Geometry: final body of the model. Coordinates: model frame, mm. Face numbers are marked on the shaded views. A direction names the side the tool comes from. Coordinates: 2 decimals unless noted, no trailing zeros. Order: outer loops, then holes, each group sorted by start corner. A loop starts at its lowest first (then second) coordinate and runs counter-clockwise, first axis right, second up. Notation, with made-up numbers: (38.25, 55) - (95.25, 55) arc R19 cw to (95.25, 71) - close; hole circle Ø2 at (7, 62.25). An arc over 180 degrees is marked (long way). Use a Markdown table: item, result. Add a question column.
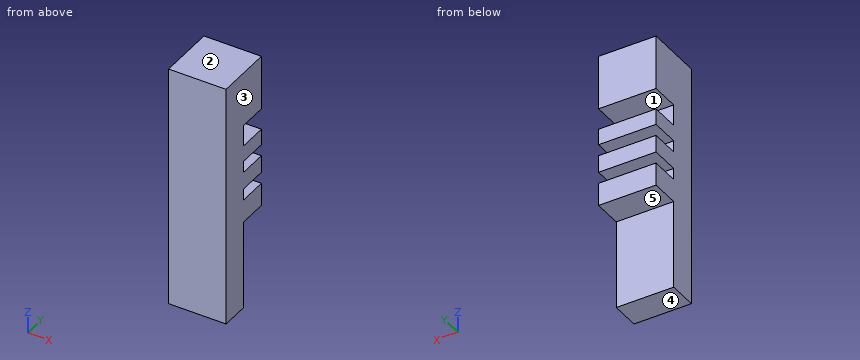
```python
from build123d import *

# Parameters (mm, degrees)
SKETCH1_W           = 10
SKETCH1_H           = 42.5
BOSS_EXTRUDE1_DEPTH = 5
SKETCH2_W           = 10
SKETCH2_H           = 4
BOSS_EXTRUDE2_DEPTH = 5


with BuildPart() as part:
    # Sketch1 → Boss-Extrude1 (new body)
    with BuildSketch(Plane(origin=(0, 0, 0), x_dir=(1, 0, 0), z_dir=(0, 1, 0))):
        with Locations((5, 21.25)):
            Rectangle(SKETCH1_W, SKETCH1_H)
    extrude(amount=BOSS_EXTRUDE1_DEPTH)

    # Sketch2 → Boss-Extrude2 (add)
    with BuildSketch(Plane(origin=(0, 5, 0), x_dir=(1, 0, 0), z_dir=(0, 1, 0))):
        with BuildLine():
            Line((0, 9.5), (0, 0))
            Line((0, 0), (10, 0))
            Line((10, 0), (10, 9.5))
            Line((10, 9.5), (6.38985528, 9.5))
            add(Edge.make_bspline(
                [(6.38985528, 9.5), (6.385913474, 9.499063167), (6.369337183, 9.495284951), (6.339528779, 9.489593982), (6.299971793, 9.48472811), (6.259281687, 9.481095847), (6.231779336, 9.480879047), (6.217848558, 9.480769231)],
                knots=[11.350502485, 11.350502485, 11.350502485, 11.350502485, 11.676244097, 12.717260333, 13.78922464, 14.880174919, 16, 16, 16, 16], degree=3))
            add(Edge.make_bspline(
                [(6.217848558, 9.480769231), (6.19658675, 9.481151208), (6.154913454, 9.481899886), (6.098774023, 9.489476712), (6.064160656, 9.496513578), (6.049680169, 9.5)],
                knots=[0, 0, 0, 0, 1.1129367, 2.181364009, 2.961379824, 2.961379824, 2.961379824, 2.961379824], degree=3))
            Line((6.049680169, 9.5), (5.326923077, 9.5))
            Line((5.326923077, 9.5), (5.192307692, 9.5))
            Line((5.192307692, 9.5), (4.903846154, 9.5))
            Line((4.903846154, 9.5), (4.769230769, 9.5))
            Line((4.769230769, 9.5), (4.12352071, 9.5))
            Line((4.12352071, 9.5), (3.942307692, 9.096153846))
            Line((3.942307692, 9.096153846), (3.796875, 9.096153846))
            Line((3.796875, 9.096153846), (3.978178742, 9.5))
            Line((3.978178742, 9.5), (3.173076923, 9.5))
            Line((3.173076923, 9.5), (3.038461538, 9.5))
            Line((3.038461538, 9.5), (2.466778357, 9.5))
            add(Edge.make_bspline(
                [(2.466778357, 9.5), (2.462836551, 9.499063167), (2.44626026, 9.495284951), (2.416451856, 9.489593982), (2.37689487, 9.48472811), (2.336204764, 9.481095847), (2.308702413, 9.480879047), (2.294771635, 9.480769231)],
                knots=[11.350502485, 11.350502485, 11.350502485, 11.350502485, 11.676244097, 12.717260333, 13.78922464, 14.880174919, 16, 16, 16, 16], degree=3))
            add(Edge.make_bspline(
                [(2.294771635, 9.480769231), (2.273509827, 9.481151208), (2.231836531, 9.481899886), (2.1756971, 9.489476712), (2.141083733, 9.496513578), (2.126603246, 9.5)],
                knots=[0, 0, 0, 0, 1.1129367, 2.181364009, 2.961379824, 2.961379824, 2.961379824, 2.961379824], degree=3))
            Line((2.126603246, 9.5), (1.5, 9.5))
            Line((1.5, 9.5), (1.353665865, 9.5))
            Line((1.353665865, 9.5), (0.223858173, 9.5))
            Line((0.223858173, 9.5), (0.076923077, 9.5))
            Line((0.076923077, 9.5), (0, 9.5))
        make_face()
        with BuildLine():
            add(Edge.make_bspline(
                [(6.38985528, 9.5), (6.385913474, 9.499063167), (6.369337183, 9.495284951), (6.339528779, 9.489593982), (6.299971793, 9.48472811), (6.259281687, 9.481095847), (6.231779336, 9.480879047), (6.217848558, 9.480769231)],
                knots=[11.350502485, 11.350502485, 11.350502485, 11.350502485, 11.676244097, 12.717260333, 13.78922464, 14.880174919, 16, 16, 16, 16], degree=3))
            Line((6.38985528, 9.5), (6.049680169, 9.5))
            add(Edge.make_bspline(
                [(6.217848558, 9.480769231), (6.19658675, 9.481151208), (6.154913454, 9.481899886), (6.098774023, 9.489476712), (6.064160656, 9.496513578), (6.049680169, 9.5)],
                knots=[0, 0, 0, 0, 1.1129367, 2.181364009, 2.961379824, 2.961379824, 2.961379824, 2.961379824], degree=3))
        make_face()
        with BuildLine():
            Line((2.466778357, 9.5), (2.126603246, 9.5))
            add(Edge.make_bspline(
                [(2.294771635, 9.480769231), (2.273509827, 9.481151208), (2.231836531, 9.481899886), (2.1756971, 9.489476712), (2.141083733, 9.496513578), (2.126603246, 9.5)],
                knots=[0, 0, 0, 0, 1.1129367, 2.181364009, 2.961379824, 2.961379824, 2.961379824, 2.961379824], degree=3))
            add(Edge.make_bspline(
                [(2.466778357, 9.5), (2.462836551, 9.499063167), (2.44626026, 9.495284951), (2.416451856, 9.489593982), (2.37689487, 9.48472811), (2.336204764, 9.481095847), (2.308702413, 9.480879047), (2.294771635, 9.480769231)],
                knots=[11.350502485, 11.350502485, 11.350502485, 11.350502485, 11.676244097, 12.717260333, 13.78922464, 14.880174919, 16, 16, 16, 16], degree=3))
        make_face()
        Polygon((3.942307692, 9.096153846), (4.12352071, 9.5), (3.978178742, 9.5), (3.796875, 9.096153846), align=None)
        with BuildLine():
            Line((0, 21), (0, 18))
            Line((0, 18), (10, 18))
            Line((10, 18), (10, 21))
            Line((10, 21), (4.598525657, 21))
            add(Edge.make_bspline(
                [(4.598525657, 21), (4.598135805, 20.999899395), (4.580997325, 20.995497464), (4.545939577, 20.988338664), (4.491951793, 20.98190012), (4.454946287, 20.981152202), (4.435997596, 20.980769231)],
                knots=[8.84081453, 8.84081453, 8.84081453, 8.84081453, 8.864066838, 9.862729781, 10.905609505, 12, 12, 12, 12], degree=3))
            add(Edge.make_bspline(
                [(4.435997596, 20.980769231), (4.414936749, 20.981260877), (4.373853136, 20.982219937), (4.320342805, 20.98961816), (4.288253752, 20.996770904), (4.275833044, 21)],
                knots=[0, 0, 0, 0, 1.145258523, 2.234067595, 2.931969346, 2.931969346, 2.931969346, 2.931969346], degree=3))
            Line((4.275833044, 21), (3.5, 21))
            Line((3.5, 21), (3.365384615, 21))
            Line((3.365384615, 21), (2.923076923, 21))
            Line((2.923076923, 21), (2.788461538, 21))
            Line((2.788461538, 21), (2.497147401, 21))
            add(Edge.make_bspline(
                [(2.497147401, 21), (2.48773707, 20.997577032), (2.45762121, 20.990585666), (2.405483538, 20.982277726), (2.362518243, 20.981276574), (2.340745192, 20.980769231)],
                knots=[5.529312578, 5.529312578, 5.529312578, 5.529312578, 5.985159533, 6.978961417, 8, 8, 8, 8], degree=3))
            add(Edge.make_bspline(
                [(2.340745192, 20.980769231), (2.321387498, 20.981294819), (2.283213267, 20.982331302), (2.232273472, 20.989625468), (2.20103719, 20.996660619), (2.188281559, 21)],
                knots=[0, 0, 0, 0, 1.033919861, 2.038935746, 2.743200613, 2.743200613, 2.743200613, 2.743200613], degree=3))
            Line((2.188281559, 21), (1.5, 21))
            Line((1.5, 21), (1.365384615, 21))
            Line((1.365384615, 21), (0.326923077, 21))
            Line((0.326923077, 21), (0.192307692, 21))
            Line((0.192307692, 21), (0, 21))
        make_face()
        with BuildLine():
            Line((0, 16), (0, 13.2))
            Line((0, 13.2), (10, 13.2))
            Line((10, 13.2), (10, 16))
            Line((10, 16), (3.521033654, 16))
            Line((3.521033654, 16), (3.115384615, 16))
            Line((3.115384615, 16), (2.418932719, 16))
            add(Edge.make_bspline(
                [(2.418932719, 16), (2.411928934, 15.997803198), (2.38964973, 15.991136542), (2.351568812, 15.981497268), (2.304119202, 15.972381089), (2.255531856, 15.966286943), (2.205701909, 15.962111836), (2.172084157, 15.961731301), (2.155048077, 15.961538462)],
                knots=[10.30831536, 10.30831536, 10.30831536, 10.30831536, 10.776456485, 11.791383307, 12.812564526, 13.85620153, 14.913611965, 16, 16, 16, 16], degree=3))
            add(Edge.make_bspline(
                [(2.155048077, 15.961538462), (2.138915077, 15.961650744), (2.107014067, 15.961872769), (2.059914602, 15.965469412), (2.014061924, 15.970376442), (1.969587085, 15.97776507), (1.926247381, 15.986484073), (1.896478302, 15.994805468), (1.881010855, 15.999495178), (1.879360723, 16)],
                knots=[0, 0, 0, 0, 1.114604814, 2.203992996, 3.262667896, 4.300477797, 5.318619304, 6.316056647, 6.435280565, 6.435280565, 6.435280565, 6.435280565], degree=3))
            Line((1.879360723, 16), (0.326923077, 16))
            Line((0.326923077, 16), (0.192307692, 16))
            Line((0.192307692, 16), (0, 16))
        make_face()
        with BuildLine():
            Line((2.418932719, 16), (1.879360723, 16))
            add(Edge.make_bspline(
                [(2.155048077, 15.961538462), (2.138915077, 15.961650744), (2.107014067, 15.961872769), (2.059914602, 15.965469412), (2.014061924, 15.970376442), (1.969587085, 15.97776507), (1.926247381, 15.986484073), (1.896478302, 15.994805468), (1.881010855, 15.999495178), (1.879360723, 16)],
                knots=[0, 0, 0, 0, 1.114604814, 2.203992996, 3.262667896, 4.300477797, 5.318619304, 6.316056647, 6.435280565, 6.435280565, 6.435280565, 6.435280565], degree=3))
            add(Edge.make_bspline(
                [(2.418932719, 16), (2.411928934, 15.997803198), (2.38964973, 15.991136542), (2.351568812, 15.981497268), (2.304119202, 15.972381089), (2.255531856, 15.966286943), (2.205701909, 15.962111836), (2.172084157, 15.961731301), (2.155048077, 15.961538462)],
                knots=[10.30831536, 10.30831536, 10.30831536, 10.30831536, 10.776456485, 11.791383307, 12.812564526, 13.85620153, 14.913611965, 16, 16, 16, 16], degree=3))
        make_face()
        with BuildLine():
            add(Edge.make_bspline(
                [(4.598525657, 21), (4.598135805, 20.999899395), (4.580997325, 20.995497464), (4.545939577, 20.988338664), (4.491951793, 20.98190012), (4.454946287, 20.981152202), (4.435997596, 20.980769231)],
                knots=[8.84081453, 8.84081453, 8.84081453, 8.84081453, 8.864066838, 9.862729781, 10.905609505, 12, 12, 12, 12], degree=3))
            Line((4.598525657, 21), (4.275833044, 21))
            add(Edge.make_bspline(
                [(4.435997596, 20.980769231), (4.414936749, 20.981260877), (4.373853136, 20.982219937), (4.320342805, 20.98961816), (4.288253752, 20.996770904), (4.275833044, 21)],
                knots=[0, 0, 0, 0, 1.145258523, 2.234067595, 2.931969346, 2.931969346, 2.931969346, 2.931969346], degree=3))
        make_face()
        with BuildLine():
            Line((2.497147401, 21), (2.188281559, 21))
            add(Edge.make_bspline(
                [(2.340745192, 20.980769231), (2.321387498, 20.981294819), (2.283213267, 20.982331302), (2.232273472, 20.989625468), (2.20103719, 20.996660619), (2.188281559, 21)],
                knots=[0, 0, 0, 0, 1.033919861, 2.038935746, 2.743200613, 2.743200613, 2.743200613, 2.743200613], degree=3))
            add(Edge.make_bspline(
                [(2.497147401, 21), (2.48773707, 20.997577032), (2.45762121, 20.990585666), (2.405483538, 20.982277726), (2.362518243, 20.981276574), (2.340745192, 20.980769231)],
                knots=[5.529312578, 5.529312578, 5.529312578, 5.529312578, 5.985159533, 6.978961417, 8, 8, 8, 8], degree=3))
        make_face()
        with Locations((5, 25)):
            Rectangle(SKETCH2_W, SKETCH2_H)
    extrude(amount=BOSS_EXTRUDE2_DEPTH)


solid = part.part
```
1) Section B-B (x = 3). Return loops of the section in (y, z).
2) Set-up query: the marked faces 4 and 5. Return all of +Z, -Z, +X, -X, +Y, -Y with unobstructed straight access to the full face (end or side cutting, diameter ignored); none if empty.
3) Section C-C (z = -36). Return loops of the section in (x, y).
4) Section A-A (y = 7.75). Return loops of the section in (x, z).
5) Pin query (flat end, axial travel): pin 1 (1.5 mm diameter, centred on x = 5, y = 6.5, fed in from +Z); pin 2 (1.6 mm diameter, centred on x = 6.5, z = -17, fed in from +Y); pin 3 (4 mm diameter, centred on x = 3, y = 8, fed in from -Z). Return the tip coordinate at first contact, or that it passes through.
6) Ray query, line 1 along Z through (x, y) = (3, 5.5); line 2 along Y through (x, z) = (4, -28.5). Return the intervals inside material, ascending.
7) Draft query along Z for the marked faces 1, 2 and 3. Return one class per face: pulls with the +Z half, pulls with the -Z half, needs draft (parallel to the pull), parting line crosses it, or undercut.
Values follow:
| question | item | result |
|---|---|---|
| 1 | outline | (0, -42.5) - (5, -42.5) - (5, -27) - (10, -27) - (10, -23) - (5, -23) - (5, -21) - (10, -21) - (10, -18) - (5, -18) - (5, -16) - (10, -16) - (10, -13.2) - (5, -13.2) - (5, -9.5) - (10, -9.5) - (10, 0) - (0, 0) - close |
| 2 | face 4 | -Z, +X, -X, +Y, -Y |
| 2 | face 5 | -Z, +X, -X, +Y |
| 3 | outline | (0, 0) - (10, 0) - (10, 5) - (0, 5) - close |
| 4 | outline | (0, -27) - (10, -27) - (10, -23) - (0, -23) - close; (0, -21) - (10, -21) - (10, -18) - (0, -18) - close; (0, -16) - (10, -16) - (10, -13.2) - (0, -13.2) - close; (0, -9.5) - (10, -9.5) - (10, 0) - (0, 0) - close |
| 5 | pin 1 | stops at z = 0 |
| 5 | pin 2 | stops at y = 5 |
| 5 | pin 3 | stops at z = -27 |
| 6 | line 1 | z = -27 to -23, -21 to -18, -16 to -13.2, -9.5 to 0 |
| 6 | line 2 | y = 0 to 5 |
| 7 | face 1 | undercut |
| 7 | face 2 | pulls with the +Z half |
| 7 | face 3 | needs draft |
